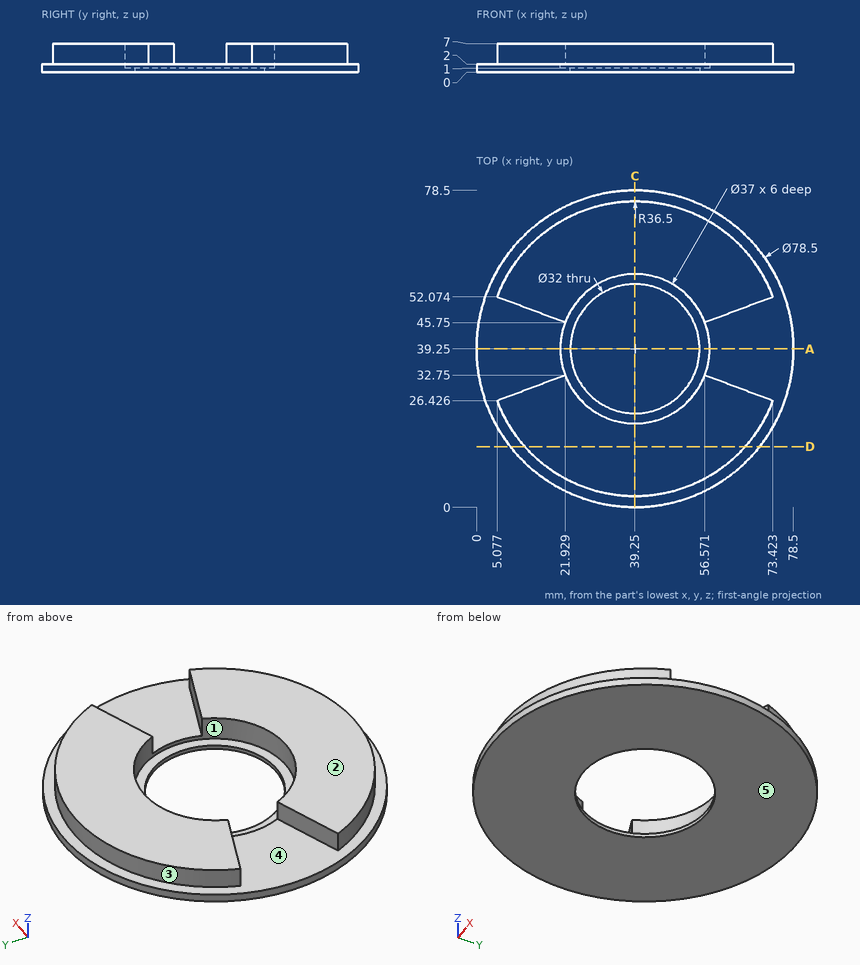
Input: dimensioned drawing with shaded views. Units: mm. Origin: part minimum x, y, z. A direction names the side the tool comes from. Give positions to 0.01 mm unless a question says otherwise; leave off trailing zeros. Loops run counter-clockwise (first coordinate to the right, second up) from the corner with the lowest first, then second, coordinate; pieces in that order, holes last. Notation, with made-up numbers: M 26,86.5 L 51,86.5 A12 ccw 51,109.5 Z; hole C 47,49 d2. An arc over 180 degrees is marked long. Put each result on its own line as item: value. Start each with the question number.
1) Contact query for a flat-ended pin moving along its axis: pin 1 (19 mm diameter, centred on x = 39.25, y = 39.25, fed in from +Z). Output: stop coordinate, or through.
2) Cut plane C-C (x = 39.25). Output: boundary loops of the cut face in (y, z).
3) Ray query, line 1 along Y through (x, z) = (39.25, 4.95); line 2 along Y through (x, z) = (9, 3) (1 decimal); line 3 along Z through (x, y) = (55, 45.5). Return the intervals inside material, ascending.
4) Pull-direction query (Y, two-part tool) for the marked faces 3, 4 and 5; classes: pulls with the +Y half, pulls with the -Y half, needs draft (parallel to the pull), parting line crosses it, or undercut.
5) Access query for the marked faces 1 and 2. Directions: +Z, -Z, +X, -X, +Y, -Y. A direction counts if a zero-diameter tool reaches every point of the face in a straight line with its end or side. Return the directions, or none.
6) Cut plane D-D (y = 15). Output: boundary loops of the cut face in (x, z), then the cut area to 3 significant figures.
7) Cut plane A-A (y = 39.25). Output: boundary loops of the cut face in (x, z).
Verdict:
1. pin 1: through
2. outline: M 0,0 L 23.25,0 L 23.25,1 L 20.75,1 L 20.75,7 L 2.75,7 L 2.75,2 L 0,2 Z; M 55.25,0 L 78.5,0 L 78.5,2 L 75.75,2 L 75.75,7 L 57.75,7 L 57.75,1 L 55.25,1 Z
3. line 1: 2.75 to 20.75, 57.75 to 75.75
3. line 2: 18.8 to 27.9, 50.6 to 59.7
3. line 3: 0 to 1
4. face 3: pulls with the +Y half
4. face 4: undercut
4. face 5: needs draft
5. face 1: +Z
5. face 2: +Z, +X, -X, +Y, -Y
6. outline: M 8.39,0 L 70.11,0 L 70.11,2 L 66.53,2 L 66.53,7 L 11.97,7 L 11.97,2 L 8.39,2 Z
6. area: 396 mm2
7. outline: M 0,0 L 23.25,0 L 23.25,1 L 20.75,1 L 20.75,2 L 0,2 Z; M 55.25,0 L 78.5,0 L 78.5,2 L 57.75,2 L 57.75,1 L 55.25,1 Z
